```python
from build123d import *

# Parameters (mm, degrees)
SKETCH3_R          = 3.175
CUT_EXTRUDE1_DEPTH = 68.57605454
FILLET1_R          = 2.54


with BuildPart() as part:
    # Sketch1 → Loft1 section 0
    with BuildSketch(Plane(origin=(0, 0, 0), x_dir=(1, 0, 0), z_dir=(0, 1, 0))):
        with BuildLine():
            Line((-53.975, -25.4), (53.975, -25.4))
            Line((53.975, -25.4), (53.975, 25.4))
            Line((53.975, 25.4), (-53.975, 25.4))
            Line((-53.975, 25.4), (-53.975, -25.4))
        make_face()
    # Sketch2 → Loft1 section 1
    with BuildSketch(Plane(origin=(0, 31.75, 0), x_dir=(1, 0, 0), z_dir=(0, 1, 0))):
        with BuildLine():
            Line((-47.625, -15.875), (47.625, -15.875))
            Line((47.625, -15.875), (47.625, 15.875))
            Line((47.625, 15.875), (-47.625, 15.875))
            Line((-47.625, 15.875), (-47.625, -15.875))
        make_face()
    loft()

    # Sketch3 → Cut-Extrude1 (cut, through all)
    with BuildSketch(Plane(origin=(0, 31.75, 0), x_dir=(1, 0, 0), z_dir=(0, 1, 0))):
        with Locations(Location((-28.575, 0, 0), (0, 0, 270))):
            Circle(SKETCH3_R)
        with Locations(Location((28.575, 0, 0), (0, 0, 90))):
            Circle(SKETCH3_R)
    extrude(amount=-CUT_EXTRUDE1_DEPTH, mode=Mode.SUBTRACT)

    # Fillet1
    fillet1_edges = [part.edges().sort_by_distance(p)[0] for p in [
        (-53.975, 0, 0),
        (0, 31.75, 15.875),
        (-47.625, 31.75, 0),
        (0, 31.75, -15.875),
        (47.625, 31.75, 0),
        (0, 0, 25.4),
        (53.975, 0, 0),
        (-50.8, 15.875, -20.6375),
        (0, 0, -25.4),
        (50.8, 15.875, -20.6375),
        (-50.8, 15.875, 20.6375),
        (50.8, 15.875, 20.6375),
    ]]
    fillet(fillet1_edges, radius=FILLET1_R)


solid = part.part
```
The model under review builds one solid part; all positions refer to its coordinate system, in mm. Give positions to 0.01 mm unless a question says otherwise; leave off trailing zeros. Answer in a Markdown table with one row per item. Add a question column.
1. Wall thickness on line 1 along X through (y, z) = (25.5, 0) (3 decimals); line 2 along X through (y, z) = (20.5, 0) (3 decimals); line 3 along Z through (x, y) = (17.5, 10): over which ranges is each line inside the solid? List them lowest first. Write a range as [from, to].
2. We need section A-A on z = 0. State how many separate pieces and enclosed holes the cut face has, then the cut area to 3 significant figures.
3. Draft analysis for pull direction Z (two halves, no side actions). For faces 1 (the cylindrical face through (25.427, 16.097, 0.413)), 2 (the flat face through (-1, 31.75, 1)), 3 (the cylindrical face through (-25.427, 16.097, -0.413)), state which applies: +Z half, -Z half, draft (parallel to the pull), parting line (faces both ways), or undercut.
4. Insertion check: P1, Ø4, axis at y = 28, z = -3, coming from the +X side (3 decimals); P2, Ø3, axis at y = 11.5, z = -12.5, coming from the +X side (3 decimals); P3, Ø1, axis at y = 4, z = -15, coming from the +X side (3 decimals); P4, Ø4, axis at x = 28.575, z = 0, coming from the +Y side. Each pin has a flat end and moves straight along its axis. Give the tip position at first contact, or say it passes through.
Ans:
| question | item | result |
|---|---|---|
| 1 | line 1 | x = [-48.875, -31.75], [-25.4, 25.4], [31.75, 48.875] |
| 1 | line 2 | x = [-49.875, -31.75], [-25.4, 25.4], [31.75, 49.875] |
| 1 | line 3 | z = [-22.4, 22.4] |
| 2 | separate pieces | 3 |
| 2 | enclosed holes | 0 |
| 2 | area | 2,820 mm^2 |
| 3 | face 1 | undercut |
| 3 | face 2 | draft |
| 3 | face 3 | undercut |
| 4 | P1 | stops at x = 48.775 |
| 4 | P2 | stops at x = 51.975 |
| 4 | P3 | stops at x = 53.275 |
| 4 | P4 | passes through |
